Design review of the part built by this model. Coordinates are the model's own, in mm. Coordinates: 2 decimals unless noted, no trailing zeros. Loops run counter-clockwise (first coordinate to the right, second up) from the corner with the lowest first, then second, coordinate; pieces in that order, holes last. Notation, with made-up numbers: (-19.5, -7.75) - (-15.5, -7.75) arc R10 ccw to (-15.5, -2.75) - close; hole circle Ø8 at (-32.75, -29.75). An arc over 180 degrees is marked (long way). Use one line per item in the form item = value. Start each with the question number.
(1) Clearance check with flat-ended pins moving along their axes: pin 1 Ø2 at (x, y) = (-25, 1) entering from +Z; pin 2 Ø3 at (y, z) = (3.5, -15) entering from +X; pin 3 Ø2 at (x, y) = (-14.5, 5) entering from +Z. State where each tip first meets the part, or that it passes through.
(2) For L1, parallel to Z at x = 0, y = 2.2; L2, parallel to Z at x = -0.5, y = 1; L3, parallel to X at y = 4.5, z = -19.5, list the stretches that pass through material, from the lowest coordinate up.
(3) Add section B-B (z = 0). State the section outline as (x, y) points, plus the area to 3 significant figures.
(4) Add section A-A (x = 0). State the section outline as (y, z) points, plus the area to 3 significant figures.
(5) Add section D-D (z = 13.5). Count the separate pieces of the cut face and the enclosed holes in it, plus the area to 3 significant figures.
(6) Add section C-C (y = 3.5). State the section outline as (x, z) points.
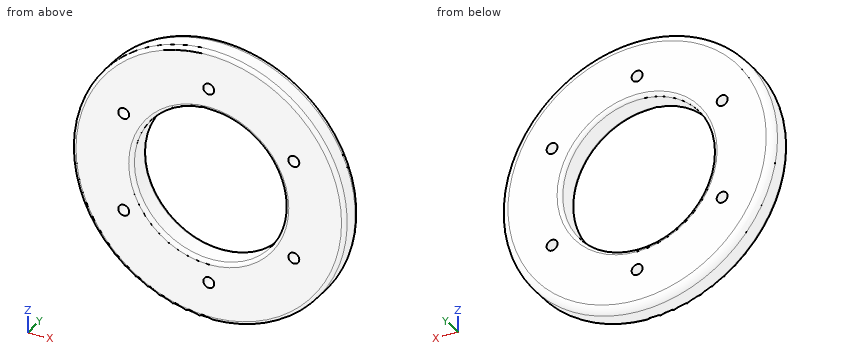
Autodesk Inventor part; units mm, degrees
ref_plane "YZ Plane" through (0, 0, 0) normal (1, 0, 0) x (0, 1, 0)
ref_plane "XZ Plane" through (0, 0, 0) normal (0, 1, 0) x (-1, 0, 0)
ref_plane "XY Plane" through (0, 0, 0) normal (0, 0, 1) x (1, 0, 0)
sketch "Esquisse1" plane through (0, 0, 0) normal (0, 1, 0) x (-1, 0, 0)
  circle A0 centre (0, 0) radius 37.5
  circle A1 centre (0, 0) radius 21
  dimension "d0" = 75
  dimension "d1" = 42
extrude "Extrusion1" add sketch "Esquisse1" along normal blind 7
fillet "Congé1" radius 2 1 edges at (37.5, 7, 0)
fillet "Congé2" radius 1 1 edges at (21, 7, 0)
fillet "Congé3" radius 1 2 edges at (37.5, 0, 0) (21, 0, 0)
sketch "Esquisse2" plane through (0, 0, 0) normal (0, -1, 0) x (1, 0, 0)
  circle A0 centre (0, 0) radius 36.5
  circle A1 centre (0, 0) radius 22
  line L0 (0, 0) -> (0, 36.5) construction
  circle A2 centre (0, 27) radius 1.5
  circle A3 centre (-23.3827, 13.5) radius 1.5
  circle A4 centre (-23.3827, -13.5) radius 1.5
  circle A5 centre (0, -27) radius 1.5
  circle A6 centre (23.3827, -13.5) radius 1.5
  circle A7 centre (23.3827, 13.5) radius 1.5
  dimension "d7" = 27
  dimension "d8" = 3
  dimension "d11" = 360
extrude "Extrusion2" cut sketch "Esquisse2" against normal through all contours A2 | A3 | A4 | A5 | A6 | A7
properties part number "encoder_wheel"
Computed values:
q1.pin_1 = 28.81
q1.pin_2 = 34.99
q1.pin_3 = 34.99
q2.L1 = -37.5 to -28.5, -25.5 to -21, 21 to 25.5, 28.5 to 37.5
q2.L2 = -37.5 to -28.41, -25.59 to -20.99, 20.99 to 25.59, 28.41 to 37.5
q2.L3 = -32.03 to -7.79, 7.79 to 32.03
q3.outline = (-37.5, 1) arc R1 ccw to (-36.5, 0) - (-22, 0) arc R1 ccw to (-21, 1) - (-21, 6) arc R1 ccw to (-22, 7) - (-35.5, 7) arc R2 ccw to (-37.5, 5) - close; (21, 1) arc R1 ccw to (22, 0) - (36.5, 0) arc R1 ccw to (37.5, 1) - (37.5, 5) arc R2 ccw to (35.5, 7) - (22, 7) arc R1 ccw to (21, 6) - close
q3.area = 228 mm^2
q4.outline = (0, -36.5) arc R1 ccw to (1, -37.5) - (5, -37.5) arc R2 ccw to (7, -35.5) - (7, -28.5) - (0, -28.5) - close; (0, -25.5) - (7, -25.5) - (7, -22) arc R1 ccw to (6, -21) - (1, -21) arc R1 ccw to (0, -22) - close; (0, 22) arc R1 ccw to (1, 21) - (6, 21) arc R1 ccw to (7, 22) - (7, 25.5) - (0, 25.5) - close; (0, 28.5) - (7, 28.5) - (7, 35.5) arc R2 ccw to (5, 37.5) - (1, 37.5) arc R1 ccw to (0, 36.5) - close
q4.area = 186 mm^2
q5.separate_pieces = 4
q5.enclosed_holes = 0
q5.area = 219 mm^2
q6.outline = circle Ø75 at (0, 0); hole circle Ø3 at (-23.38, -13.5); hole circle Ø3 at (-23.38, 13.5); hole circle Ø42 at (0, 0); hole circle Ø3 at (0, -27); hole circle Ø3 at (0, 27); hole circle Ø3 at (23.38, -13.5); hole circle Ø3 at (23.38, 13.5)
